```python
from build123d import *

# Parameters (mm, degrees)
SKETCH2_R               = 2.85
CUT_EXTRUDE1_DEPTH      = 10
CHAMFER1_SIZE           = 1
SKETCH4_R               = 1.5
BOSS_EXTRUDE1_DEPTH     = 6
CUT_EXTRUDE2_DEPTH      = 25.489997958
CUT_EXTRUDE2_DEPTH_BACK = 25.489997958
BOSS_EXTRUDE2_DEPTH     = 1.5
FILLET1_R               = 1.5
SKETCH7_R               = 0.6
CUT_EXTRUDE3_DEPTH      = 3


with BuildPart() as part:
    # Sketch1 → Revolve1 (revolve)
    with BuildSketch(Plane(origin=(0, 0, 0), x_dir=(1, 0, 0), z_dir=(0, 1, 0))):
        Polygon((0, 0), (0, 7), (2, 7), (2, 6), (12.4, 6), (12.4, 5.5), (16.4, 5.5), (16.4, 0), align=None)
    revolve(axis=Axis((16.4, 0, 0), (-1, 0, 0)))

    # Sketch2 → Cut-Extrude1 (cut)
    with BuildSketch(Plane.ZY):
        Circle(SKETCH2_R)
    extrude(amount=-CUT_EXTRUDE1_DEPTH, mode=Mode.SUBTRACT)

    # Chamfer1
    chamfer1_edges = [part.edges().sort_by_distance(p)[0] for p in [
        (0, 0, -2.85),
    ]]
    chamfer(chamfer1_edges, length=CHAMFER1_SIZE)

    # Sketch4 → Boss-Extrude1 (add)
    with BuildSketch(Plane(origin=(16.4, 0, 0), x_dir=(0, 0, -1), z_dir=(1, 0, 0))):
        Circle(SKETCH4_R)
    extrude(amount=BOSS_EXTRUDE1_DEPTH)

    # Sketch5 → Cut-Extrude2 (cut, two sides: drawn at the far end of the back side and taken through both)
    with BuildSketch(Plane(origin=(0, 0, 0), x_dir=(1, 0, 0), z_dir=(0, 1, 0)).offset(-CUT_EXTRUDE2_DEPTH_BACK)):
        Polygon((22.4, -1.5), (19.4, -1.5), (19.4, -0.5), (22.4, 0), align=None)
    extrude(amount=CUT_EXTRUDE2_DEPTH + CUT_EXTRUDE2_DEPTH_BACK, mode=Mode.SUBTRACT)

    # Sketch6 → Boss-Extrude2 (add, symmetric)
    with BuildSketch(Plane(origin=(0, 0, 0), x_dir=(1, 0, 0), z_dir=(0, 1, 0))):
        Polygon((16.4, 5), (26.1, 5.848640036), (26.143577871, 5.350542687), (16.4, 4.498090081), align=None)
    extrude(amount=BOSS_EXTRUDE2_DEPTH, both=True)

    # Fillet1
    fillet1_edges = [part.edges().sort_by_distance(p)[0] for p in [
        (26.121788936, 1.5, -5.599591362),
        (26.121788936, -1.5, -5.599591362),
    ]]
    fillet(fillet1_edges, radius=FILLET1_R - 0.0001)  # a hair under: the kernel refuses the full size

    # Sketch7 → Cut-Extrude3 (cut)
    with BuildSketch(Plane(origin=(-0.309544019, 0, -3.538104326), x_dir=(-0.9961946980917462, 0, 0.08715574274765167), z_dir=(-0.08715574274765167, 0, -0.9961946980917462))):
        with Locations((-25.010424187, 0)):
            Circle(SKETCH7_R)
    extrude(amount=-CUT_EXTRUDE3_DEPTH, mode=Mode.SUBTRACT)


solid = part.part
```
Geometry check sheet. Reference: the model listing, model coordinates, mm. A direction names the side the tool comes from. Give positions to 0.01 mm unless a question says otherwise; leave off trailing zeros. Order: outer loops, then holes, each group sorted by start corner. A loop starts at its lowest first (then second) coordinate and runs counter-clockwise, first axis right, second up. Notation, with made-up numbers: (43.25, 5.25) - (99.25, 5.25) arc R9 ccw to (99.25, 22.25) - close; hole circle Ø5 at (11, 42.25). An arc over 180 degrees is marked (long way). Write item = value, one per line. Start each with the question number.
1) Section check C-C (z = 4.5). Enter the section's corners in (x, y).
2) Access from +Z, -Z, +X, -X, +Y, -Y to the whole of each face (thin tool, end or side, straight path). Record for faces 4 (the cylindrical face through (18.69, 0.45, -1.43)), 5 (the flat face through (22.4, 0, -1)), 6 (the cylindrical face through (5.437, -1.734, -2.262)).
3) Section check B-B (y = 5). Enter the section's corners in (x, z), then the cut area to 3 significant figures.
4) Section check A-A (x = 18.75). Enter the section's corners in (y, z), then the cut area to 3 significant figures.
5) Section check D-D (x = 16). Enter the section's corners in (y, z).
6) Draft check along Z on faces 1 (the flat face through (19.4, 0, 1)), 2 (the flat face through (21.34, 0.02, -4.93)), 3 (the cylindrical face through (25.224, 0.026, -5.525)). Enter one of: released by +Z, released by -Z, zero draft, split by the parting line, or undercut.
7) Scan lines: L1, parallel to Y at x = 4.75, z = 0; L2, parallel to X at y = 5.25, z = -0.25; L3, parallel to X at y = -4, z = 5.5. Record each from-to range of solid material in increasing order.
8) Gauge pin test, flat ends, axial feed: pin 1 Ø6.5 at (y, z) = (0, 0) entering from -X; pin 2 Ø1.7 at (y, z) = (-0.5, 1) entering from -X; pin 3 Ø2 at (y, z) = (-2.5, -1) entering from +X. Record the tip position at first contact, or that the pin passes through.
Geometry check:
q1.outline = (0, -5.36) - (2, -5.36) - (2, -3.97) - (12.4, -3.97) - (12.4, -3.16) - (16.4, -3.16) - (16.4, 3.16) - (12.4, 3.16) - (12.4, 3.97) - (2, 3.97) - (2, 5.36) - (0, 5.36) - close
q2.face_4 = +X
q2.face_5 = +Z, +X, +Y, -Y
q2.face_6 = -X
q3.outline = (0, -4.9) - (2, -4.9) - (2, -3.32) - (12.4, -3.32) - (12.4, -2.29) - (16.4, -2.29) - (16.4, 2.29) - (12.4, 2.29) - (12.4, 3.32) - (2, 3.32) - (2, 4.9) - (0, 4.9) - close
q3.area = 107 mm2
q4.outline = (-1.5, -5.21) - (1.5, -5.21) - (1.5, -4.7) - (-1.5, -4.7) - close; circle Ø3 at (0, 0)
q4.area = 8.57 mm2
q5.outline = circle Ø11 at (0, 0)
q6.face_1 = zero draft
q6.face_2 = undercut
q6.face_3 = split by the parting line
q7.L1 = -6 to -2.85, 2.85 to 6
q7.L2 = 0 to 16.4
q7.L3 = 0 to 2
q8.pin_1 = 0.6
q8.pin_2 = 10
q8.pin_3 = 16.4
